Part print with two shaded views. Sizes in mm from the minimum x, y, z corner. Round coordinates to 2 decimals unless told otherwise and drop trailing zeros. Write each loop counter-clockwise with the first axis right and the second up, starting at its lowest first coordinate (ties: lowest second). Pieces come first, ordered by that corner, then holes. Notation, with made-up numbers: (7, 36.5) -> (24, 36.5) arc R21 cw to (24, 63.5) -> close; hole circle Ø7 at (43, -3). An arc over 180 degrees is marked (long way). Return JSON: item names as keys, results as strings. Group by question number.
(1) Saw through at B-B (z = 52). List the corners of the cut face in (x, y), plus the area to 3 significant figures.
(2) Drill centre lines: L1, parallel to Y at x = 4.15, z = 53.5; L2, parallel to Z at x = 2.7, y = 13. Where is each one in solid material? Low to high. Write a range as from..to.
(3) Saw through at A-A (x = 1.1). List the corners of the cut face in (y, z).
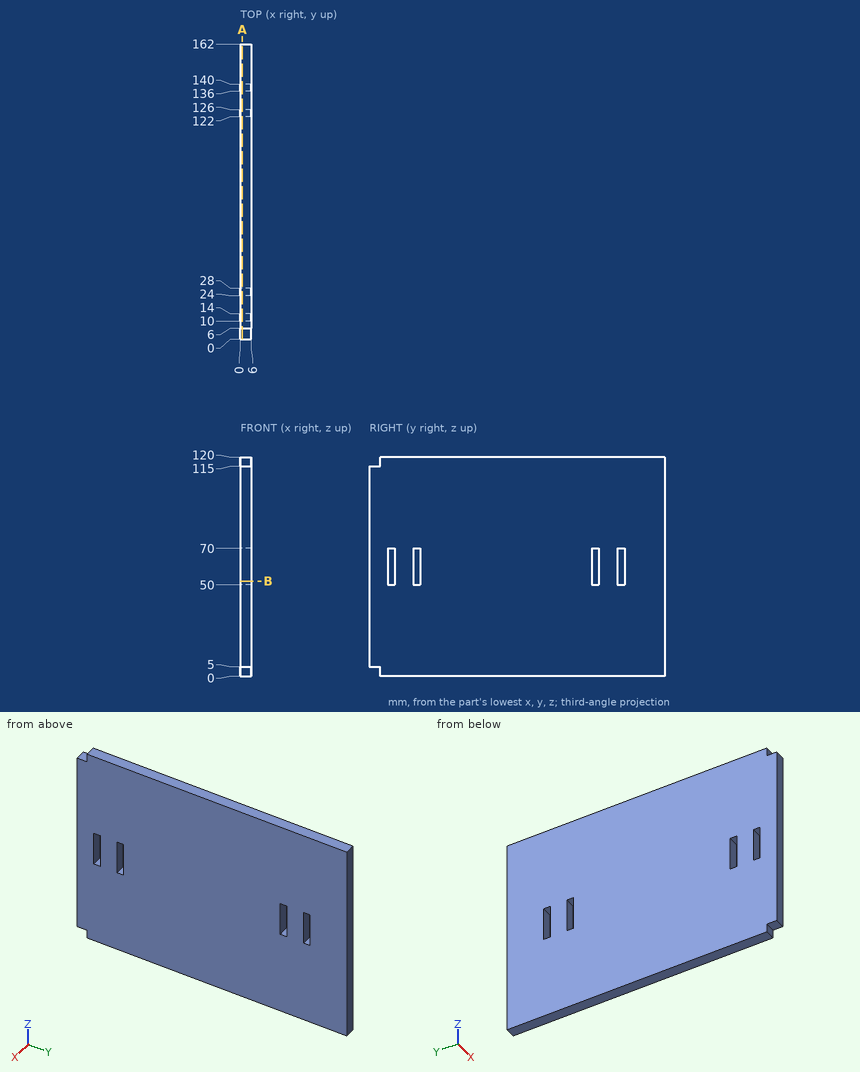
Computed values:
{
 "1": {"outline": "(0, 0) -> (6, 0) -> (6, 10) -> (0, 10) -> close; (0, 14) -> (6, 14) -> (6, 24) -> (0, 24) -> close; (0, 28) -> (6, 28) -> (6, 122) -> (0, 122) -> close; (0, 126) -> (6, 126) -> (6, 136) -> (0, 136) -> close; (0, 140) -> (6, 140) -> (6, 162) -> (0, 162) -> close", "area": "876 mm2"},
 "2": {"L1": "0..10, 14..24, 28..122, 126..136, 140..162", "L2": "0..50, 70..120"},
 "3": {"outline": "(0, 5) -> (6, 5) -> (6, 0) -> (162, 0) -> (162, 120) -> (6, 120) -> (6, 115) -> (0, 115) -> close; hole (10, 50) -> (14, 50) -> (14, 70) -> (10, 70) -> close; hole (24, 50) -> (28, 50) -> (28, 70) -> (24, 70) -> close; hole (122, 50) -> (126, 50) -> (126, 70) -> (122, 70) -> close; hole (136, 50) -> (140, 50) -> (140, 70) -> (136, 70) -> close"}
}
